For this review, take the finished solid that the model builds, in its own axes (mm). Coordinates: 2 decimals unless noted, no trailing zeros. Loops run counter-clockwise (first coordinate to the right, second up) from the corner with the lowest first, then second, coordinate; pieces in that order, holes last.
1. Clearance check with a flat-ended pin moving along its axis: P1, Ø15.5, axis at x = 0, z = -50, coming from the +Y side. State where the tip first meets the part, or that it passes through.
2. Mouldability with a two-part tool opening along Z and no side actions: class faces 1 (the face through (-50, 0, -1)), 2 (the face through (-5.745, 0.056, -43.735)), 3 (the face through (1, 0, -70)) as pulls with the +Z half, pulls with the -Z half, needs draft (parallel to the pull), parting line crosses it, or undercut.
3. To check wall thickness, follow probe 1 along Z at (x, y) = (0, 1.25); probe 2 along X at (y, z) = (-0.5, 50); probe 3 along X at (y, z) = (0.5, 57.5). State the ranges of each line that lie inside material, in increasing order.
4. Take a section at B-B, the plane x = 0. State the section outline as (y, z) points.
5. Take a section at D-D, the plane z = 53. State the section outline as (x, y) points.
6. Take a section at C-C, the plane y = 1.5. State the section outline as (x, z) points, then the cut area to 3 significant figures.
7. Take a section at A-A, the plane z = -50. State the section outline as (x, y) points.
Autodesk Inventor part; units mm, degrees
ref_plane "YZ Plane" through (0, 0, 0) normal (1, 0, 0) x (0, 1, 0)
ref_plane "XZ Plane" through (0, 0, 0) normal (0, 1, 0) x (-1, 0, 0)
ref_plane "XY Plane" through (0, 0, 0) normal (0, 0, 1) x (1, 0, 0)
sketch "Sketch1" plane through (0, 0, 0) normal (0, 1, 0) x (-1, 0, 0)
  line L0 (50, 70) -> (-50, 70)
  line L1 (-50, 70) -> (-50, -70)
  line L2 (-50, -70) -> (50, -70)
  line L3 (50, -70) -> (50, 70)
  point P0 (0, 0)
  point P1 (0, 70)
  point P2 (50, 0)
  dimension "d0" = 100
  dimension "d1" = 140
extrude "Plate1" add sketch "Sketch1" along normal mid plane 8
sketch "Sketch2" plane through (0, -4, 0) normal (0, -1, 0) x (1, 0, 0)
  line L0 (-50, -70) -> (-50, 70)
  line L1 (50, 70) -> (50, -70)
  line L2 (0, -50) -> (0, 50) construction
  point P0 (-50, 0)
  point P1 (0, 0)
  point P2 (0, 0)
  dimension "d17" = 100
hole "Hole1" at (0, -4, -50) at (0, -4, 50) direction (0, 1, 0) diameter 17 end through all
fillet "Fillet1" radius 2 4 edges at (50, 0, 70) (-50, 0, 70) (50, 0, -70) (-50, 0, -70)
equation "\"d8\" = Thickness"
equation "\"d2\" = Thickness"
equation "\"BendRadius\" = Thickness"
equation "\"BendReliefWidth\" = Thickness"
equation "\"BendReliefDepth\" = 0.5 * Thickness"
equation "\"CornerReliefSize\" = 4 * Thickness"
equation "\"MinimumRemnant\" = 2 * Thickness"
equation "\"TransitionRadius\" = BendRadius"
equation "\"JacobiRadiusSize\" = BendRadius"
equation "\"GapSize\" = Thickness"
properties part number "Сrane plate 5.1"
Results list:
1. P1: passes through
2. face 1: needs draft
2. face 2: undercut
2. face 3: pulls with the -Z half
3. probe 1: z = -70 to -58.5, -41.5 to 41.5, 58.5 to 70
3. probe 2: x = -50 to -8.5, 8.5 to 50
3. probe 3: x = -50 to -4, 4 to 50
4. outline: (-4, -70) - (4, -70) - (4, -58.5) - (-4, -58.5) - close; (-4, -41.5) - (4, -41.5) - (4, 41.5) - (-4, 41.5) - close; (-4, 58.5) - (4, 58.5) - (4, 70) - (-4, 70) - close
5. outline: (-50, -4) - (-7.95, -4) - (-7.95, 4) - (-50, 4) - close; (7.95, -4) - (50, -4) - (50, 4) - (7.95, 4) - close
6. outline: (-50, -68) arc R2 ccw to (-48, -70) - (48, -70) arc R2 ccw to (50, -68) - (50, 68) arc R2 ccw to (48, 70) - (-48, 70) arc R2 ccw to (-50, 68) - close; hole circle Ø17 at (0, -50); hole circle Ø17 at (0, 50)
6. area: 13,500 mm2
7. outline: (-50, -4) - (-8.5, -4) - (-8.5, 4) - (-50, 4) - close; (8.5, -4) - (50, -4) - (50, 4) - (8.5, 4) - close
